Autodesk Fusion 360 part; units mm, degrees
sketch "Sketch1" plane through (0, 0, 0) normal (0, 0, 1) x (1, 0, 0) in component "Component'"
  line L0 (-39.5, 0) -> (39.5, 0)
  line L1 (-39.5, 0) -> (-39.5, -2)
  line L2 (-39.5, -2) -> (-41.5, -2)
  line L3 (-41.5, -2) -> (-41.5, -3)
  line L4 (0, 0) -> (0, -5.5) construction
  line L5 (39.5, 0) -> (39.5, -2)
  line L6 (39.5, -2) -> (41.5, -2)
  line L7 (41.5, -2) -> (41.5, -3)
  line L8 (-41.5, -3) -> (41.5, -3)
  line L9 (-27.5, -5.5) -> (27.5, -5.5)
  line L10 (27.5, -5.5) -> (27.5, -3)
  line L11 (-27.5, -5.5) -> (-27.5, -3)
  line L12 (-39.5, -2) -> (-39.5, -3)
  line L13 (39.5, -2) -> (39.5, -3)
  dimension "d19" = 79
  dimension "d20" = 2
  dimension "d21" = 2
  dimension "d22" = 1
  dimension "d23" = 5.5
  dimension "d24" = 55
extrude "Extrude1" add sketch "Sketch1" along normal blind 15 contours L0 L1 L5 L8 L12 L13 | L8 L9 L10 L11 in component "Component'"
extrude "Extrude2" add sketch "Sketch1" along normal blind 6 contours L2 L3 L8 L12 | L6 L7 L8 L13 in component "Component'"
sketch "Sketch2" plane through (0, -5.5, 0) normal (0, -1, 0) x (1, 0, 0) in component "Component'"
  line L0 (-27.5, 0) -> (27.5, 0)
  line L1 (27.5, 0) -> (27.5, 15)
  line L2 (27.5, 15) -> (-27.5, 15)
  line L3 (-27.5, 15) -> (-27.5, 0)
  line L4 (-25.5, 13) -> (-14.5, 13)
  line L5 (-14.5, 13) -> (-14.5, 2)
  line L6 (-14.5, 2) -> (-25.5, 2)
  line L7 (-25.5, 2) -> (-25.5, 13)
  line L8 (-27.5, 0) -> (27.5, 0)
  line L9 (0, 0) -> (0, 15) construction
  line L10 (25.5, 13) -> (14.5, 13)
  line L11 (25.5, 2) -> (25.5, 13)
  line L12 (14.5, 13) -> (14.5, 2)
  line L13 (14.5, 2) -> (25.5, 2)
  dimension "d29" = 11
  dimension "d30" = 11
  dimension "d31" = 2
  dimension "d32" = 2
extrude "Extrude3" cut sketch "Sketch2" against normal up to surface (5.5 mm away) contours L4 L5 L6 L7 | L10 L11 L12 L13 in component "Component'"
sketch "Sketch3" plane through (0, 0, 15) normal (0, 0, 1) x (-1, 0, 0) in component "Component'"
  line L0 (39.5, 0) -> (39.5, 3)
  line L1 (39.5, 3) -> (27.5, 3)
  line L2 (27.5, 3) -> (27.5, 5.5)
  line L3 (27.5, 5.5) -> (-27.5, 5.5)
  line L4 (-27.5, 5.5) -> (-27.5, 3)
  line L5 (-27.5, 3) -> (-39.5, 3)
  line L6 (-39.5, 3) -> (-39.5, 0)
  line L7 (-39.5, 0) -> (39.5, 0)
  line L8 (39.5, 0.3) -> (-39.5, 0.3)
  line L9 (27.5, 5.2) -> (-27.5, 5.2)
  line L10 (39.5, 0) -> (-39.5, 0)
  line L11 (27.5, 5.5) -> (-27.5, 5.5)
  dimension "d36" = 0.3
  dimension "d37" = 0.3
extrude "Extrude4" add sketch "Sketch3" against normal up to surface (15 mm away) contours L0 L6 L7 L8 L10 | L2 L3 L4 L9 L11 in component "Component'"
component "Component'" placed x (1, 0, 0) y (0, 1, 0) z (0, 0, 1) at (0, 0, 0)
Geometry: final body of the model. Coordinates: model frame, mm. A direction names the side the tool comes from. Coordinates: 2 decimals unless noted, no trailing zeros. Order: outer loops, then holes, each group sorted by start corner. A loop starts at its lowest first (then second) coordinate and runs counter-clockwise, first axis right, second up.
(1) Section query C-C (y = -4.25). Return the cut outline in (x, z).
(2) Section query A-A (x = -17). Return the cut outline in (y, z), plus the area to 3 significant figures.
(3) Access query for faces 1 (the face through (-40, -2, 3)), 2 (the face through (14.5, -3, 8)), 3 (the face through (-1, -3, 15)). Directions: +Z, -Z, +X, -X, +Y, -Y. A direction counts if a zero-diameter tool reaches every point of the face in a straight line with its end or side. Return the directions, or none.
(4) Draft query along Y for faces 4 (the face through (34, -3, 7)), 5 (the face through (-27.5, -4, 7)), 6 (the face through (-20, -3, 13)), 7 (the face through (-20, -5.2, 8)). Return one class per face: pulls with the +Y half, pulls with the -Y half, needs draft (parallel to the pull), parting line crosses it, or undercut.
(5) Material intervals for probe 1 along X at (y, z) = (-1.5, 6.25); probe 2 along X at (y, z) = (-4.05, 12.25); probe 3 along Y at (x, z) = (23, 12.75), sorted ascending.
(6) Section query D-D (z = 14). Return the cut outline in (x, y), plus the area to 4 significant figures.
(7) Section query B-B (z = 3.25). Return the cut outline in (x, y), plus the area to 3 significant figures.
(8) First-contact query: pin 1 (1.5 mm diameter, centred on y = -1.5, z = 7.5, fed in from -X); pin 2 (4 mm diameter, centred on x = 37.5, z = 8.5, fed in from -Y); pin 3 (1.6 mm diameter, centred on x = 40.5, z = 4, fed in from +Y). Flat tips, straight axial feed; report the tip coordinate or a pass-through.
Solution:
1. outline: (-27.5, 0) - (27.5, 0) - (27.5, 15) - (-27.5, 15) - close; hole (-25.5, 2) - (-14.5, 2) - (-14.5, 13) - (-25.5, 13) - close; hole (14.5, 2) - (25.5, 2) - (25.5, 13) - (14.5, 13) - close
2. outline: (-5.5, 0) - (0, 0) - (0, 15) - (-5.5, 15) - close; hole (-5.2, 2) - (-0.3, 2) - (-0.3, 13) - (-5.2, 13) - close
2. area: 28.6 mm2
3. face 1: +Z, -Z, -X, +Y
3. face 2: none
3. face 3: +Z, +X, -X, +Y, -Y
4. face 4: pulls with the -Y half
4. face 5: needs draft
4. face 6: undercut
4. face 7: undercut
5. probe 1: x = -39.5 to -25.5, -14.5 to 14.5, 25.5 to 39.5
5. probe 2: x = -27.5 to -25.5, -14.5 to 14.5, 25.5 to 27.5
5. probe 3: y = -5.5 to -5.2, -0.3 to 0
6. outline: (-39.5, -3) - (-27.5, -3) - (-27.5, -5.5) - (27.5, -5.5) - (27.5, -3) - (39.5, -3) - (39.5, 0) - (-39.5, 0) - close
6. area: 374.5 mm2
7. outline: (-41.5, -3) - (-27.5, -3) - (-27.5, -5.5) - (27.5, -5.5) - (27.5, -3) - (41.5, -3) - (41.5, -2) - (39.5, -2) - (39.5, 0) - (-39.5, 0) - (-39.5, -2) - (-41.5, -2) - close; hole (-25.5, -5.2) - (-14.5, -5.2) - (-14.5, -0.3) - (-25.5, -0.3) - close; hole (14.5, -5.2) - (25.5, -5.2) - (25.5, -0.3) - (14.5, -0.3) - close
7. area: 271 mm2
8. pin 1: stops at x = -39.5
8. pin 2: stops at y = -3
8. pin 3: stops at y = -2
